The model under review builds one solid part; all positions refer to its coordinate system, in mm. Coordinates: 2 decimals unless noted, no trailing zeros. Write each loop counter-clockwise with the first axis right and the second up, starting at its lowest first coordinate (ties: lowest second). Pieces come first, ordered by that corner, then holes.
1) For P1, Ø2, axis at y = 66, z = 59, coming from the -X side; P2, Ø1.5, axis at x = -240.5, y = -52, coming from the +Z side; P3, Ø0.8, axis at x = -249.5, y = 94.5, coming from the +Z side, all flat-tipped, find the tip position at first contact; note any pin that passes through.
2) For line 1 (Y direction, x = -240.25, z = 364); line 2 (X direction, y = -272, z = 338); line 3 (Z direction, x = -243.75, y = 108), list the stretches that pass through material, from the lowest coordinate up.
3) Add section C-C, the plane y = -74. State the section outline as (x, z) points.
4) Add section B-B, the plane x = -243.5. State the section outline as (y, z) points, then the cut area to 3 significant figures.
5) Add section A-A, the plane z = 41. State the section outline as (x, y) points, then the cut area to 3 significant figures.
from build123d import *

# Parameters (mm, degrees)
CROQUIS1_W              = 500
CROQUIS1_H              = 700
SALIENTE_EXTRUIR1_DEPTH = 500
VACIADO1_T              = -1
CROQUIS2_W              = 15
CROQUIS2_H              = 20
SALIENTE_EXTRUIR2_DEPTH = 2
SALIENTE_EXTRUIR3_START = -20
CROQUIS3_R              = 3
SALIENTE_EXTRUIR3_DEPTH = 20
SALIENTE_EXTRUIR4_START = -20
SALIENTE_EXTRUIR4_DEPTH = 20
CORTAR_EXTRUIR1_DEPTH   = 792.853048236
CROQUIS6_R              = 797.844751534
CORTAR_EXTRUIR2_DEPTH   = 50
CROQUIS7_W              = 449
CROQUIS7_H              = 499
CORTAR_EXTRUIR3_DEPTH   = 50
CROQUIS8_W              = 449
CROQUIS8_H              = 699
CORTAR_EXTRUIR4_DEPTH   = 50
CROQUIS9_W              = 449
CROQUIS9_H              = 500
CORTAR_EXTRUIR5_DEPTH   = 50
SALIENTE_EXTRUIR5_DEPTH = 10


with BuildPart() as part:
    # Croquis1 → Saliente-Extruir1 (new body)
    with BuildSketch(Plane.XY):
        Rectangle(CROQUIS1_W, CROQUIS1_H)
    extrude(amount=SALIENTE_EXTRUIR1_DEPTH)

    # Vaciado1
    vaciado1_openings = [part.faces().sort_by_distance(p)[0] for p in [
        (0, 0, 500),
    ]]
    offset(amount=VACIADO1_T, openings=vaciado1_openings, kind=Kind.INTERSECTION)

    # Croquis2 → Saliente-Extruir2 (add)
    with BuildSketch(Plane(origin=(-249, 0, 0), x_dir=(0, 0, -1), z_dir=(1, 0, 0))):
        with Locations((-492.5, 220)):
            Rectangle(CROQUIS2_W, CROQUIS2_H)
        with Locations((-492.5, -220)):
            Rectangle(CROQUIS2_W, CROQUIS2_H)
    extrude(amount=SALIENTE_EXTRUIR2_DEPTH)

    # Croquis3 → Saliente-Extruir3 (add)
    with BuildSketch(Plane.XZ.offset(230).offset(SALIENTE_EXTRUIR3_START)):
        with Locations((-248.5, 502.5)):
            Circle(CROQUIS3_R)
    extrude(amount=SALIENTE_EXTRUIR3_DEPTH)

    # Croquis4 → Saliente-Extruir4 (add)
    with BuildSketch(Plane.XZ.offset(-210).offset(SALIENTE_EXTRUIR4_START)):
        with BuildLine():
            Line((-250, 499.901923789), (-247, 499.901923789))
            ThreePointArc((-247, 499.901923789), (-248.5, 505.5), (-250, 499.901923789))
        make_face()
    extrude(amount=SALIENTE_EXTRUIR4_DEPTH)

    # Croquis5 → Cortar-Extruir1 (cut, through all)
    with BuildSketch(Plane(origin=(-249, 0, 0), x_dir=(0, 0, -1), z_dir=(1, 0, 0))):
        Polygon((-485, -210), (-485, -230), (-500, -230), (-500, -349), (-1, -349), (-1, 349), (-500, 349), (-500, 230), (-485, 230), (-485, 210), (-500, 210), (-500, -210), align=None)
    extrude(amount=CORTAR_EXTRUIR1_DEPTH, mode=Mode.SUBTRACT)


with BuildPart() as cortar_extruir1_piece_1:
    # of the separate pieces the step leaves, piece 1, a body of its own (cortar_extruir1_pieces)
    add(part.part.solids().sort_by_distance((-250, -350, 0))[0])


with BuildPart() as cortar_extruir1_piece_2:
    # of the separate pieces the step leaves, piece 2, a body of its own (cortar_extruir1_pieces)
    add(part.part.solids().sort_by_distance((250, 210, 500))[0])


with BuildPart() as cortar_extruir1_piece_3:
    # of the separate pieces the step leaves, piece 3, a body of its own (cortar_extruir1_pieces)
    add(part.part.solids().sort_by_distance((250, -230, 485))[0])


with BuildPart() as cortar_extruir2_tool:
    # Croquis6 → Cortar-Extruir2 (new body)
    with BuildSketch(Plane(origin=(250, 0, 0), x_dir=(0, 0, -1), z_dir=(1, 0, 0))):
        with Locations((-1, 0)):
            Circle(CROQUIS6_R)
    extrude(amount=-CORTAR_EXTRUIR2_DEPTH)


with BuildPart() as cortar_extruir1_piece_1_1:
    add(cortar_extruir1_piece_1.part)

    # Cortar-Extruir2: cut by cortar_extruir2_tool
    add(cortar_extruir2_tool.part, mode=Mode.SUBTRACT)

    # Croquis7 → Cortar-Extruir3 (cut)
    with BuildSketch(Plane(origin=(0, -349, 0), x_dir=(1, 0, 0), z_dir=(0, 1, 0))):
        with Locations((-24.5, -250.5)):
            Rectangle(CROQUIS7_W, CROQUIS7_H)
    extrude(amount=-CORTAR_EXTRUIR3_DEPTH, mode=Mode.SUBTRACT)

    # Croquis8 → Cortar-Extruir4 (cut)
    with BuildSketch(Plane.XY.offset(1)):
        with Locations((-24.5, -0.5)):
            Rectangle(CROQUIS8_W, CROQUIS8_H)
    extrude(amount=-CORTAR_EXTRUIR4_DEPTH, mode=Mode.SUBTRACT)

    # Croquis9 → Cortar-Extruir5 (cut)
    with BuildSketch(Plane.XZ.offset(-349)):
        with Locations((-24.5, 250)):
            Rectangle(CROQUIS9_W, CROQUIS9_H)
    extrude(amount=-CORTAR_EXTRUIR5_DEPTH, mode=Mode.SUBTRACT)

    # Croquis10 → Saliente-Extruir5 (add)
    with BuildSketch(Plane(origin=(-249, 0, 0), x_dir=(0, 0, -1), z_dir=(1, 0, 0))):
        Polygon((2, -352), (2, 352), (-502, 352), (-502, 350), (-500, 350), (-499, 349), (-1, 349), (-1, -349), (-499, -349), (-500, -350), (-502, -350), (-502, -352), align=None)
    extrude(amount=SALIENTE_EXTRUIR5_DEPTH)


with BuildPart() as cortar_extruir1_piece_2_1:
    add(cortar_extruir1_piece_2.part)

    # Cortar-Extruir2: cut by cortar_extruir2_tool
    add(cortar_extruir2_tool.part, mode=Mode.SUBTRACT)


with BuildPart() as cortar_extruir1_piece_3_1:
    add(cortar_extruir1_piece_3.part)

    # Cortar-Extruir2: cut by cortar_extruir2_tool
    add(cortar_extruir2_tool.part, mode=Mode.SUBTRACT)


solid = cortar_extruir1_piece_1_1.part
Geometry results:
1. P1: stops at x = -250
1. P2: stops at z = 1
1. P3: stops at z = 500
2. line 1: y = -352 to -349, 349 to 352
2. line 2: x = -250 to -249
2. line 3: z = -2 to 1
3. outline: (-250, 0) - (-249, 0) - (-249, -2) - (-239, -2) - (-239, 1) - (-249, 1) - (-249, 500) - (-250, 500) - close
4. outline: (-352, -2) - (352, -2) - (352, 502) - (350, 502) - (350, 500) - (349, 499) - (349, 1) - (-349, 1) - (-349, 499) - (-350, 500) - (-350, 502) - (-352, 502) - close
4. area: 5,110 mm2
5. outline: (-250, -350) - (-249, -350) - (-249, -352) - (-239, -352) - (-239, -349) - (-249, -349) - (-249, 349) - (-239, 349) - (-239, 352) - (-249, 352) - (-249, 350) - (-250, 350) - close
5. area: 760 mm2
